Design review of the part shown in the three views and the two pictorial views. Dimensions are in mm from the part's minimum x, y and z. A direction names the side the tool comes from. Round coordinates to 2 decimals unless told otherwise and drop trailing zeros. Loops run counter-clockwise (first coordinate to the right, second up) from the corner with the lowest first, then second, coordinate; pieces in that order, holes last. Notation, with made-up numbers: (25, 62.5) - (30, 62.5) arc R10 ccw to (30, 74.5) - close; hole circle Ø4 at (61, 49). An arc over 180 degrees is marked (long way). Return JSON: item names as keys, results as strings. Group by question number.
(1) We need section D-D, the plane x = 3.75. Write out the cut boundary in (y, z) (3 decimals), and give its area (3 significant figures).
(2) We need section C-C, the plane y = 11. Write out the cut boundary in (x, z) (3 decimals), and give its area (3 significant figures).
(3) We need section B-B, the plane y = 3. Write out the cut boundary in (x, z) (3 decimals), and give its area (3 significant figures).
(4) Wall thickness on L1, parallel to X at y = 29, z = 5.45; L2, parallel to Z at x = 9.5, y = 28 (3 decimals): over which ranges is each line inside the solid? List them lowest first. Write a range as [from, to].
(5) For the marked faces 4 and 5, list the 3-axis set-ups (+Z, -Z, +X, -X, +Y, -Y) from which the entire face can be reached by the end or side of a thin tool; tool diameter is ignored.
(6) The part is to be moulded in two halves that separate along X. For the marked faces 1, 2 and 3, say which applies: pulls with the +X half, pulls with the -X half, needs draft (parallel to the pull), parting line crosses it, or undercut.
(7) We need section A-A, the plane z = 3.75. Write out the cut boundary in (x, y).
(8) Clearance check with flat-ended pins moving along their axes: pin 1 (10 mm diameter, centred on x = 10, y = 17.5, fed in from +Z) (3 decimals); pin 2 (0.5 mm diameter, centred on x = 16, z = 0.5, fed in from -Y); pin 3 (2 mm diameter, centred on x = 10, y = 22, fed in from -Z). State where each tip first meets the part, or that it passes through.
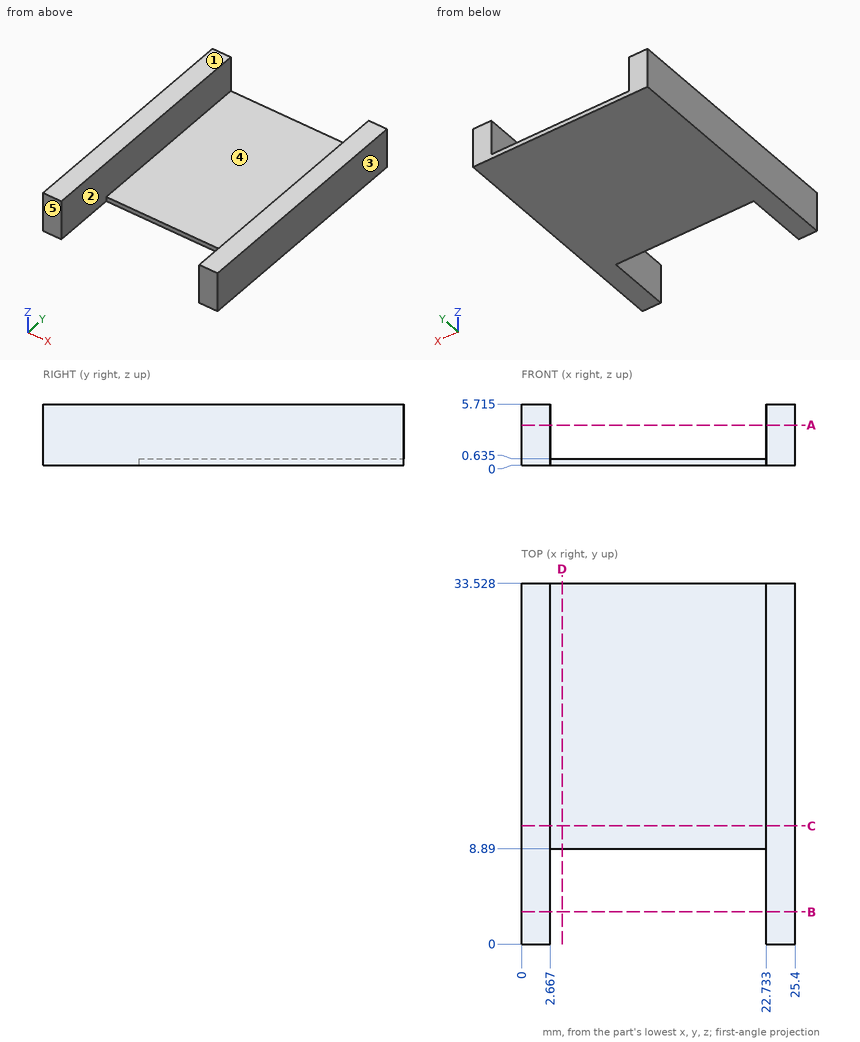
Solutions:
{
 "1": {"outline": "(8.89, 0) - (33.528, 0) - (33.528, 0.635) - (8.89, 0.635) - close", "area": "15.6 mm^2"},
 "2": {"outline": "(0, 0) - (25.4, 0) - (25.4, 5.715) - (22.733, 5.715) - (22.733, 0.635) - (2.667, 0.635) - (2.667, 5.715) - (0, 5.715) - close", "area": "43.2 mm^2"},
 "3": {"outline": "(0, 0) - (2.667, 0) - (2.667, 5.715) - (0, 5.715) - close; (22.733, 0) - (25.4, 0) - (25.4, 5.715) - (22.733, 5.715) - close", "area": "30.5 mm^2"},
 "4": {"L1": "[0, 2.67], [22.73, 25.4]", "L2": "[0, 0.635]"},
 "5": {"face 4": "+Z, +Y, -Y", "face 5": "+Z, -Z, +X, -X, -Y"},
 "6": {"face 1": "needs draft", "face 2": "undercut", "face 3": "pulls with the +X half"},
 "7": {"outline": "(0, 0) - (2.67, 0) - (2.67, 33.53) - (0, 33.53) - close; (22.73, 0) - (25.4, 0) - (25.4, 33.53) - (22.73, 33.53) - close"},
 "8": {"pin 1": "z = 0.635", "pin 2": "y = 8.89", "pin 3": "z = 0"}
}
